from build123d import *

# Parameters (mm, degrees)
SKETCH1_R           = 60.325
BOSS_EXTRUDE1_DEPTH = 10
SKETCH2_R           = 13.49375
BOSS_EXTRUDE2_DEPTH = 117
CUT_EXTRUDE1_START  = -28.1
SKETCH3_R           = 13.49375
CUT_EXTRUDE1_DEPTH  = 28.1
SKETCH4_R           = 8.449063039
BOSS_EXTRUDE3_DEPTH = 28.1


with BuildPart() as part:
    # Sketch1 → Boss-Extrude1 (new body)
    with BuildSketch(Plane.XY):
        Circle(SKETCH1_R)
    extrude(amount=BOSS_EXTRUDE1_DEPTH)

    # Sketch2 → Boss-Extrude2 (add)
    with BuildSketch(Plane.XY.offset(10)):
        Circle(SKETCH2_R)
    extrude(amount=BOSS_EXTRUDE2_DEPTH)

    # Sketch3 → Cut-Extrude1 (cut)
    with BuildSketch(Plane.XY.offset(127).offset(CUT_EXTRUDE1_START)):
        Circle(SKETCH3_R)
    extrude(amount=CUT_EXTRUDE1_DEPTH, mode=Mode.SUBTRACT)

    # Sketch4 → Boss-Extrude3 (add)
    with BuildSketch(Plane.XY.offset(98.9)):
        Circle(SKETCH4_R)
    extrude(amount=BOSS_EXTRUDE3_DEPTH)


solid = part.part
Can you work these out from the model? Positions are in its coordinate system, mm. A direction names the side the tool comes from. Round coordinates to 2 decimals unless told otherwise and drop trailing zeros. Loops run counter-clockwise (first coordinate to the right, second up) from the corner with the lowest first, then second, coordinate; pieces in that order, holes last. Notation, with made-up numbers: (32, -7) - (37, -7) arc R27 ccw to (37, 21) - close; hole circle Ø11 at (75.5, 29). An arc over 180 degrees is marked (long way). Answer in a Markdown table with one row per item. Add a question column.
Q1. I want a section at C-C on z = 107. List the corners of the cut face in (x, y) for me, and give its area (3 significant figures).
Q2. I want a section at D-D on z = 21.5. List the corners of the cut face in (x, y) for me.
Q3. I want a section at A-A on y = 0. List the corners of the cut face in (x, z) for me (3 decimals).
Q4. I need wall thicknesses on L1, parallel to Z at x = -23.5, y = -49.5; L2, parallel to Y at x = -0.5, z = 70; L3, parallel to Y at x = -2, z = 82. Which ranges of each line are inside material? Lowest first, please.
Q5. For pin 1 Ø5 at (y, z) = (6, 19) entering from +X; pin 2 Ø5 at (x, y) = (-37.5, -36.5) entering from +Z, each with a flat end and sliding along its axis, tell me the tip position at first contact or that it passes through.
Q6. Which directions (+Z, -Z, +X, -X, +Y, -Y) give clear straight access to the entire face, cutting with the end or side of a thin tool? Please do faces 1 (the cylindrical face through (-60.267, 2.652, 4.93)), 2 (the cylindrical face through (-1.1, 8.377, 112.753)).
A:
| question | item | result |
|---|---|---|
| 1 | outline | circle Ø16.9 at (0, 0) |
| 1 | area | 224 mm^2 |
| 2 | outline | circle Ø26.99 at (0, 0) |
| 3 | outline | (-60.325, 0) - (60.325, 0) - (60.325, 10) - (13.494, 10) - (13.494, 98.9) - (8.449, 98.9) - (8.449, 127) - (-8.449, 127) - (-8.449, 98.9) - (-13.494, 98.9) - (-13.494, 10) - (-60.325, 10) - close |
| 4 | L1 | 0 to 10 |
| 4 | L2 | -13.48 to 13.48 |
| 4 | L3 | -13.34 to 13.34 |
| 5 | pin 1 | x = 13.03 |
| 5 | pin 2 | z = 10 |
| 6 | face 1 | +Z, -Z |
| 6 | face 2 | +Z |
